CAD build for the part. Positions are in the model's coordinates, mm. A direction names the side the tool comes from. Round coordinates to 2 decimals unless told otherwise and drop trailing zeros. Order: outer loops, then holes, each group sorted by start corner. A loop starts at its lowest first (then second) coordinate and runs counter-clockwise, first axis right, second up. Notation, with made-up numbers: M 41,-39 L 71,-39 A21 cw 71,-34 Z; hole C 8.5,-35 d10. An arc over 180 degrees is marked long. Answer as a JSON object with one key per item and string values.
```python
from build123d import *

# Parameters (mm, degrees)
SKETCH5_W            = 80
SKETCH5_H            = 90
BOSS_EXTRUDE2_DEPTH  = 1.5
M4_CLEARANCE_HOLE2_D = 4.5
SKETCH8_R            = 38
CUT_EXTRUDE1_DEPTH   = 2
BOSS_EXTRUDE3_DEPTH  = 1.5
SKETCH10_W           = 2
SKETCH10_H           = 59.5
BOSS_EXTRUDE4_DEPTH  = 1.5


with BuildPart() as part:
    # Sketch5 → Boss-Extrude2 (new body)
    with BuildSketch(Plane.XY):
        Rectangle(SKETCH5_W, SKETCH5_H)
    extrude(amount=BOSS_EXTRUDE2_DEPTH)

    # M4 Clearance Hole2 (through all)
    with Locations(Plane.XY.offset(1.5)):
        with Locations((35.75, 35.75), (-35.75, -35.75), (-35.75, 35.75), (35.75, -35.75)):
            Hole(M4_CLEARANCE_HOLE2_D / 2)

    # Sketch8 → Cut-Extrude1 (cut)
    with BuildSketch(Plane.XY.offset(1.5)):
        Circle(SKETCH8_R)
    extrude(amount=-CUT_EXTRUDE1_DEPTH, mode=Mode.SUBTRACT)

    # Sketch9 → Boss-Extrude3 (add)
    with BuildSketch(Plane.XY.offset(1.5)):
        with BuildLine():
            Line((-18.828232369, 33.007539531), (-33.007539531, 18.828232369))
            ThreePointArc((-33.007539531, 18.828232369), (-34.372809901, 16.202158483), (-35.52955283, 13.477791945))
            Line((-35.52955283, 13.477791945), (-13.477791945, 35.52955283))
            ThreePointArc((-13.477791945, 35.52955283), (-16.202158483, 34.372809901), (-18.828232369, 33.007539531))
        make_face()
        with BuildLine():
            Line((-4.052476159, 37.78329574), (-37.78329574, 4.052476159))
            ThreePointArc((-37.78329574, 4.052476159), (-37.915095853, 2.538800193), (-37.986279438, 1.021065336))
            Line((-37.986279438, 1.021065336), (-1.021065336, 37.986279438))
            ThreePointArc((-1.021065336, 37.986279438), (-2.538800193, 37.915095853), (-4.052476159, 37.78329574))
        make_face()
        with BuildLine():
            Line((5.729767662, 37.565539561), (-37.565539561, -5.729767662))
            ThreePointArc((-37.565539561, -5.729767662), (-37.363427276, -6.926348402), (-37.123210121, -8.115865346))
            Line((-37.123210121, -8.115865346), (8.115865346, 37.123210121))
            ThreePointArc((8.115865346, 37.123210121), (6.926348402, 37.363427276), (5.729767662, 37.565539561))
        make_face()
        with BuildLine():
            Line((13.634094956, 35.469866855), (-35.469866855, -13.634094956))
            ThreePointArc((-35.469866855, -13.634094956), (-35.067590884, -14.637761769), (-34.636921504, -15.629576729))
            Line((-34.636921504, -15.629576729), (15.629576729, 34.636921504))
            ThreePointArc((15.629576729, 34.636921504), (14.637761769, 35.067590884), (13.634094956, 35.469866855))
        make_face()
        with BuildLine():
            Line((20.292391155, 32.128163054), (-32.128163054, -20.292391155))
            ThreePointArc((-32.128163054, -20.292391155), (-31.572249627, -21.146939577), (-30.993612648, -21.986267874))
            Line((-30.993612648, -21.986267874), (21.986267874, 30.993612648))
            ThreePointArc((21.986267874, 30.993612648), (21.146939577, 31.572249627), (20.292391155, 32.128163054))
        make_face()
        with BuildLine():
            Line((25.936489585, 27.772261485), (-27.772261485, -25.936489585))
            ThreePointArc((-27.772261485, -25.936489585), (-27.080082578, -26.658378187), (-26.369145748, -27.361800973))
            Line((-26.369145748, -27.361800973), (27.361800973, 26.369145748))
            ThreePointArc((27.361800973, 26.369145748), (26.658378187, 27.080082578), (25.936489585, 27.772261485))
        make_face()
        with BuildLine():
            Line((30.64028313, 22.47605503), (-22.47605503, -30.64028313))
            ThreePointArc((-22.47605503, -30.64028313), (-21.648561438, -31.230430475), (-20.805580736, -31.798235961))
            Line((-20.805580736, -31.798235961), (31.798235961, 20.805580736))
            ThreePointArc((31.798235961, 20.805580736), (31.230430475, 21.648561438), (30.64028313, 22.47605503))
        make_face()
        with BuildLine():
            Line((34.370751902, 16.206523801), (-16.206523801, -34.370751902))
            ThreePointArc((-16.206523801, -34.370751902), (-15.228749713, -34.815013747), (-14.238811494, -35.23146672))
            Line((-14.238811494, -35.23146672), (35.23146672, 14.238811494))
            ThreePointArc((35.23146672, 14.238811494), (34.815013747, 15.228749713), (34.370751902, 16.206523801))
        make_face()
        with BuildLine():
            Line((36.966476918, 8.802248818), (-8.802248818, -36.966476918))
            ThreePointArc((-8.802248818, -36.966476918), (-7.632453052, -37.225604903), (-6.455069393, -37.447724619))
            Line((-6.455069393, -37.447724619), (37.447724619, 6.455069393))
            ThreePointArc((37.447724619, 6.455069393), (37.225604903, 7.632453052), (36.966476918, 8.802248818))
        make_face()
        with BuildLine():
            Line((37.999643576, -0.164584524), (0.164584524, -37.999643576))
            ThreePointArc((0.164584524, -37.999643576), (1.644059958, -37.964418432), (3.121041877, -37.871613348))
            Line((3.121041877, -37.871613348), (37.871613348, -3.121041877))
            ThreePointArc((37.871613348, -3.121041877), (37.964418432, -1.644059958), (37.999643576, -0.164584524))
        make_face()
        with BuildLine():
            Line((36.000661901, -12.1635662), (12.1635662, -36.000661901))
            ThreePointArc((12.1635662, -36.000661901), (14.624168706, -35.073261748), (17.014742957, -33.977912268))
            Line((17.014742957, -33.977912268), (33.977912268, -17.014742957))
            ThreePointArc((33.977912268, -17.014742957), (35.073261748, -14.624168706), (36.000661901, -12.1635662))
        make_face()
    extrude(amount=-BOSS_EXTRUDE3_DEPTH)

    # Sketch10 → Boss-Extrude4 (add)
    with BuildSketch(Plane(origin=(0, 0, 0), x_dir=(-1, 0, 0), z_dir=(0, 0, -1))):
        with Locations((-39, 0)):
            Rectangle(SKETCH10_W, SKETCH10_H)
        with Locations((39, 0)):
            Rectangle(SKETCH10_W, SKETCH10_H)
    extrude(amount=BOSS_EXTRUDE4_DEPTH)


solid = part.part
```
Item 1: Saw through at A-A on x = 28.5. List the corners of the cut face in (y, z).
Worked answers:
{"outline": "M -45,0 L -25.13,0 L -25.13,1.5 L -45,1.5 Z; M -22.49,0 L -19.66,0 L -19.66,1.5 L -22.49,1.5 Z; M -12.49,0 L -9.66,0 L -9.66,1.5 L -12.49,1.5 Z; M -2.49,0 L 0.34,0 L 0.34,1.5 L -2.49,1.5 Z; M 7.51,0 L 10.34,0 L 10.34,1.5 L 7.51,1.5 Z; M 17.51,0 L 20.34,0 L 20.34,1.5 L 17.51,1.5 Z; M 25.13,0 L 45,0 L 45,1.5 L 25.13,1.5 Z"}
Item 2: 3-axis set-ups, long thin cutter, end or side, ignore diameter. For faces 4 (the flat face through (39, 0, -1.5)), 5 (the flat face through (-14.82, 14.19, 0.76)): which of +Z, -Z, +X, -X, +Y, -Y reach the whole face in a straight line?
Worked answers:
{"face 4": "-Z, +X, -X, +Y, -Y", "face 5": "+Z, -Z"}
Item 3: Saw through at B-B on y = 3. State how many separate pieces and enclosed holes the cut face has, and give its area (3 significant figures).
Worked answers:
{"separate pieces": "9", "enclosed holes": "0", "area": "44.9 mm2"}
Item 4: Wall check: line 1 along X through (y, z) = (-1.5, -0.85); line 2 along Y through (x, z) = (32, 1); line 3 along X through (y, z) = (-32, 0.9). Give the ranges that are in metal, low to high. Write a range as [from, to].
Worked answers:
{"line 1": "x = [-40, -38], [38, 40]", "line 2": "y = [-45, -20.49], [-18.99, -16.16], [-8.99, -6.16], [1.01, 3.84], [11.01, 13.84], [20.49, 45]", "line 3": "x = [-40, -20.49], [-13.84, -11.01], [-3.84, -1.01], [6.16, 8.99], [16.16, 18.99], [20.49, 40]"}
Item 5: Drop flat-ended pins along their axis: pin 1 Ø6 at (x, y) = (-15, 30) entering from -Z; pin 2 Ø1.2 at (x, z) = (38.5, -1) entering from -Y; pin 3 Ø12 at (x, y) = (1, -31) entering from +Z; pin 4 Ø3.5 at (x, y) = (-35.75, -35.75) entering from +Z. Give the stop position or say it passes through.
Worked answers:
{"pin 1": "stops at z = 0", "pin 2": "stops at y = -29.75", "pin 3": "stops at z = 1.5", "pin 4": "passes through"}
Item 6: Two-plate mould, pull along X, no slides. Class faces 1 (the flat face through (40, -1, 0)), 2 (the cylindrical face through (33.18, 18.52, 0.76)), 3 (the flat face through (-39, 0, -1.5)): released by +X, released by -X, zero draft, split by the parting line, or undercut.
Worked answers:
{"face 1": "released by +X", "face 2": "undercut", "face 3": "zero draft"}
